Model file for the job. Use its own axes, mm. Face numbers are marked on the shaded views. A direction names the side the tool comes from. Round coordinates to 2 decimals unless told otherwise and drop trailing zeros. Write each loop counter-clockwise with the first axis right and the second up, starting at its lowest first coordinate (ties: lowest second). Pieces come first, ordered by that corner, then holes.
```python
from build123d import *

# Parameters (mm, degrees)
SKETCH1_W           = 25.4
SKETCH1_H           = 25.4
SKETCH1_R           = 4.7625
BOSS_EXTRUDE1_DEPTH = 25.4
CHAMFER1_SIZE       = 1.27
SKETCH3_R           = 4.7625
CUT_EXTRUDE1_DEPTH  = 26.4


with BuildPart() as part:
    # Sketch1 → Boss-Extrude1 (new body)
    with BuildSketch(Plane(origin=(0, 0, 0), x_dir=(1, 0, 0), z_dir=(0, 1, 0))):
        Rectangle(SKETCH1_W, SKETCH1_H)
        Circle(SKETCH1_R, mode=Mode.SUBTRACT)
    extrude(amount=BOSS_EXTRUDE1_DEPTH)

    # Chamfer1
    chamfer1_edges = [part.edges().sort_by_distance(p)[0] for p in [
        (-4.7625, 0, 0),
        (-4.7625, 25.4, 0),
    ]]
    chamfer(chamfer1_edges, length=CHAMFER1_SIZE)

    # Sketch2 → Revolve1 (revolve)
    with BuildSketch(Plane(origin=(0, 12.7, 0), x_dir=(1, 0, 0), z_dir=(0, 1, 0))):
        with BuildLine():
            Line((-36.83, -3.175), (36.83, -3.175))
            Line((36.83, -3.175), (36.83, -5.715))
            ThreePointArc((36.83, -5.715), (40.871115254, -4.041115254), (42.545, 0))
            Line((42.545, 0), (-42.545, 0))
            ThreePointArc((-42.545, 0), (-40.871115254, -4.041115254), (-36.83, -5.715))
            Line((-36.83, -5.715), (-36.83, -3.175))
        make_face()
    revolve(axis=Axis((-42.545, 12.7, 0), (1, 0, 0)))

    # Sketch3 → Cut-Extrude1 (cut, through all)
    with BuildSketch(Plane(origin=(0, 25.4, 0), x_dir=(1, 0, 0), z_dir=(0, 1, 0))):
        Circle(SKETCH3_R)
    extrude(amount=-CUT_EXTRUDE1_DEPTH, mode=Mode.SUBTRACT)


solid = part.part
```
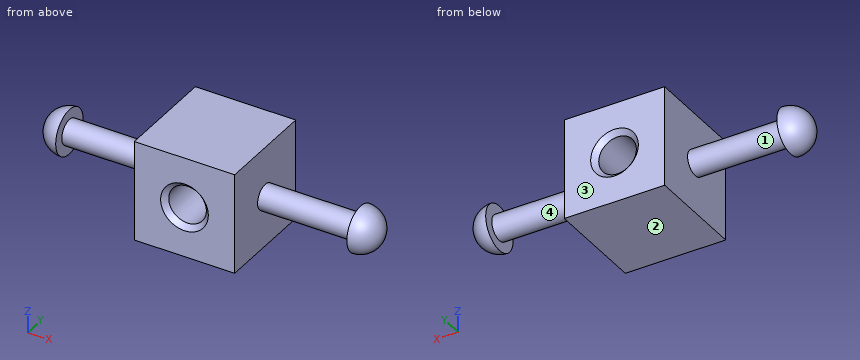
1) Wall check: probe 1 along X at (y, z) = (16.75, 0); probe 2 along X at (y, z) = (3.75, 0.25); probe 3 along Z at (x, y) = (23.5, 13). Give the ranges that are in metal, low to high.
2) Cut at B-B on x = 0. List the corners of the cut face in (y, z).
3) Which spindle directions (+Z, -Z, +X, -X, +Y, -Y) get a long thin tool onto all of the face, cutting with end or side? Do the marked faces 1 and 2. Say none if no direction does.
4) Pull direction X, two halves, no side cores. Call the marked faces 3 and 4: released by +X, released by -X, zero draft, split by the parting line, or undercut.
5) Cut at C-C on y = 7.75. List the corners of the cut face in (x, z) (1 decimal), and give its area (3 significant figures).
6) Flat gauge pins, fed straight in: pin 1 Ø3.5 at (y, z) = (11, -1) entering from -X; pin 2 Ø2 at (y, z) = (10, -9.5) entering from +X; pin 3 Ø11 at (x, z) = (0, 0) entering from +Y. Where does each tip first touch, or does it go through?
7) Cut at A-A on z = 0. List the corners of the cut face in (x, y) (1 decimal), and give its area (3 significant figures).
Result sheet:
1. probe 1: x = -40.86 to -36.83, -12.7 to -4.76, 4.76 to 12.7, 36.83 to 40.86
1. probe 2: x = -12.7 to -4.76, 4.76 to 12.7
1. probe 3: z = -3.16 to 3.16
2. outline: (0, -12.7) - (25.4, -12.7) - (25.4, -6.03) - (24.13, -4.76) - (1.27, -4.76) - (0, -6.03) - close; (0, 6.03) - (1.27, 4.76) - (24.13, 4.76) - (25.4, 6.03) - (25.4, 12.7) - (0, 12.7) - close
3. face 1: none
3. face 2: -Z, +X, -X, +Y, -Y
4. face 3: zero draft
4. face 4: undercut
5. outline: (-36.8, -2.9) - (-36.8, 2.9) arc R2.9 ccw to start; (-12.7, -12.7) - (12.7, -12.7) - (12.7, 12.7) - (-12.7, 12.7) - close; (36.8, -2.9) arc R2.9 ccw to (36.8, 2.9) - close; hole circle Ø9.5 at (0, 0)
5. area: 600 mm2
6. pin 1: stops at x = -42.54
6. pin 2: stops at x = 12.7
6. pin 3: stops at y = 24.87
7. outline: (-36.8, 7) - (-36.8, 9.5) - (-12.7, 9.5) - (-12.7, 0) - (-6, 0) - (-4.8, 1.3) - (-4.8, 24.1) - (-6, 25.4) - (-12.7, 25.4) - (-12.7, 15.9) - (-36.8, 15.9) - (-36.8, 18.4) arc R5.7 ccw to start; (4.8, 1.3) - (6, 0) - (12.7, 0) - (12.7, 9.5) - (36.8, 9.5) - (36.8, 7) arc R5.7 ccw to (36.8, 18.4) - (36.8, 15.9) - (12.7, 15.9) - (12.7, 25.4) - (6, 25.4) - (4.8, 24.1) - close
7. area: 809 mm2
